Source: three-view drawing plus pictorial views. Frame: mm from the lowest corner of the part. A direction names the side the tool comes from. Give positions to 0.01 mm unless a question says otherwise; leave off trailing zeros. Order: outer loops, then holes, each group sorted by start corner. A loop starts at its lowest first (then second) coordinate and runs counter-clockwise, first axis right, second up.
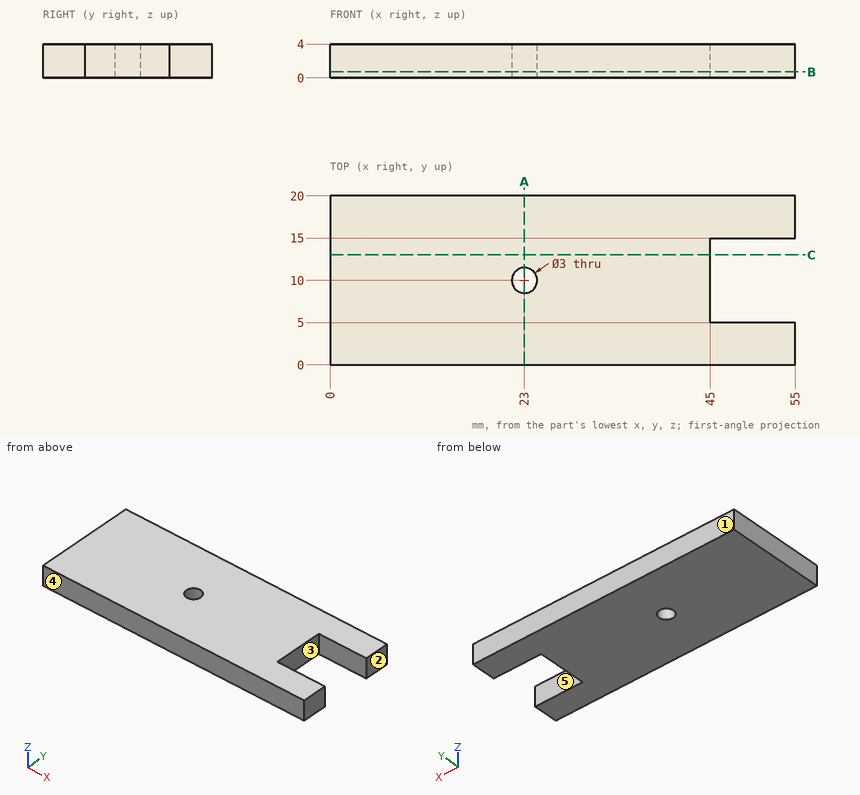
(1) Pin query (flat end, axial travel): pin 1 Ø1.2 at (y, z) = (11.5, 1) entering from +X. Return the tip coordinate at first contact, or that it passes through.
(2) Line query: line 1 along Y through (x, z) = (53, 1.9); line 2 along Y through (x, z) = (23, 1.25); line 3 along X through (y, z) = (14.25, 2.85). Output: solid intervals per line, ascending.
(3) Section B-B, the plane z = 0.7. Return loops of the section in (x, y).
(4) Access query for the marked faces 4 and 5. Directions: +Z, -Z, +X, -X, +Y, -Y. A direction counts if a zero-diameter tool reaches every point of the face in a straight line with its end or side. Return the directions, or none.
(5) Section C-C, the plane y = 13. Return loops of the section in (x, z), plus the area to 3 significant figures.
(6) Draft query along Y for the marked faces 1, 2 and 3. Return one class per face: +Y half, -Y half, draft (parallel to the pull), parting line (faces both ways), or undercut.
(7) Section A-A, the plane x = 23. Return loops of the section in (y, z).
Checks:
1. pin 1: stops at x = 45
2. line 1: y = 0 to 5, 15 to 20
2. line 2: y = 0 to 8.5, 11.5 to 20
2. line 3: x = 0 to 45
3. outline: (0, 0) - (55, 0) - (55, 5) - (45, 5) - (45, 15) - (55, 15) - (55, 20) - (0, 20) - close; hole circle Ø3 at (23, 10)
4. face 4: +Z, -Z, +X, -X, -Y
4. face 5: +Z, -Z, +X
5. outline: (0, 0) - (45, 0) - (45, 4) - (0, 4) - close
5. area: 180 mm2
6. face 1: +Y half
6. face 2: draft
6. face 3: undercut
7. outline: (0, 0) - (8.5, 0) - (8.5, 4) - (0, 4) - close; (11.5, 0) - (20, 0) - (20, 4) - (11.5, 4) - close
